```python
from build123d import *

# Parameters (mm, degrees)
F0_R         = 25
F1_DEPTH     = 60
F2_W         = 33.9622593881
F2_H         = 36.695571085
F3_DEPTH     = 25
F4_R         = 18.3477855425
F5_DEPTH     = 25.0000003725
F6_R         = 5
F8_T1_DEPTH  = 37.8584149398
F8_T6_ANGLE  = 94.4306250519
F8_T11_ANGLE = 94.4306250519
F8_T16_ANGLE = 94.4306250519
F8_T21_ANGLE = 47.2153125259
F8_T26_ANGLE = 47.2153125259
F8_T31_ANGLE = 47.2153125259
F8_T36_ANGLE = 47.2153125259
F8_T41_ANGLE = 85.5693749481
F8_T46_ANGLE = 85.5693749481
F8_T51_ANGLE = 85.5693749481
F8_T56_ANGLE = 85.5693749481
F8_T61_ANGLE = 85.5693749481
F8_T66_ANGLE = 85.5693749481
F9_R         = 14.0953649679
F10_DEPTH    = 200


# Not quite as in the source:
# - a fillet or chamfer that OpenCascade refuses, or shapes differently, is made with other operations: its cross-section is extruded or revolved along the edge and cut away or added
# - a feature of the source that left no trace in its solid (it failed there, or was rolled back) is left out


with BuildPart() as f1:
    # F0 (on Front) → F1 (new body)
    with BuildSketch(Plane.XZ):
        Circle(F0_R)
    extrude(amount=F1_DEPTH)

    # F2 (on face) → F3 (join)
    with BuildSketch(Plane.XZ.offset(60)):
        Rectangle(F2_W, F2_H)
    extrude(amount=F3_DEPTH)

    # F4 (on face) → F5 (join)
    with BuildSketch(Plane.XZ.offset(85)):
        Circle(F4_R)
    extrude(amount=F5_DEPTH)

    # F6
    f6_edges = [f1.edges().sort_by_distance(p)[0] for p in [
        (-18.347786, -110, 0),
    ]]
    fillet(f6_edges, radius=F6_R)

    # F8: chamfer of 5 on 9 edges, made by hand

    # F8_s2 → F8_t1 (cut)
    with BuildSketch(Plane.XZ.offset(60)):
        Polygon((16.9811296941, -13.3477855425), (11.9811296941, -18.3477855425), (16.9811296941, -18.3477855425), align=None)
        Polygon((16.9811296941, 13.3477855425), (11.9811296941, 18.3477855425), (16.9811296941, 18.3477855425), align=None)
        Polygon((-11.9811296941, -18.3477855425), (-16.9811296941, -13.3477855425), (-16.9811296941, -18.3477855425), align=None)
        Polygon((-16.9811296941, 13.3477855425), (-11.9811296941, 18.3477855425), (-16.9811296941, 18.3477855425), align=None)
    extrude(amount=F8_T1_DEPTH, mode=Mode.SUBTRACT)


with BuildPart() as f8_tool4:
    # F8_s5 → F8_t6 (revolve)
    with BuildSketch(Plane(origin=(0, 0, 0), x_dir=(0, 1, 0), z_dir=(0.7339114217, 0, 0.6792451878))):
        Polygon((-60, 20), (-55, 25), (-60, 25), align=None)
    revolve(axis=Axis((0, -60, 0), (0, -1, 0)), revolution_arc=F8_T6_ANGLE)

    split(bisect_by=Plane(origin=(-15.1644576183, 0, 15.1644576183), x_dir=(0, 1, 0), z_dir=(-0.7071067812, 0, 0.7071067812)), keep=Keep.TOP)


with BuildPart() as f1_1:
    add(f1.part)

    # F8_t3: cut F8_tool4
    add(f8_tool4.part, mode=Mode.SUBTRACT)


with BuildPart() as f8_tool9:
    # F8_s10 → F8_t11 (revolve)
    with BuildSketch(Plane(origin=(0, 0, 0), x_dir=(0, 1, 0), z_dir=(0.7339114217, 0, 0.6792451878))):
        Polygon((-60, 20), (-55, 25), (-60, 25), align=None)
    revolve(axis=Axis((0, -60, 0), (0, -1, 0)), revolution_arc=F8_T11_ANGLE)

    split(bisect_by=Plane.YZ.offset(-16.9811296941), keep=Keep.BOTTOM)


with BuildPart() as f1_2:
    add(f1_1.part)

    # F8_t8: cut F8_tool9
    add(f8_tool9.part, mode=Mode.SUBTRACT)


with BuildPart() as f8_tool14:
    # F8_s15 → F8_t16 (revolve)
    with BuildSketch(Plane(origin=(0, 0, 0), x_dir=(0, 1, 0), z_dir=(0.7339114217, 0, 0.6792451878))):
        Polygon((-60, 20), (-55, 25), (-60, 25), align=None)
    revolve(axis=Axis((0, -60, 0), (0, -1, 0)), revolution_arc=F8_T16_ANGLE)

    split(bisect_by=Plane(origin=(-15.1644576183, 0, -15.1644576183), x_dir=(0, 1, 0), z_dir=(-0.7071067812, 0, -0.7071067812)), keep=Keep.TOP)


with BuildPart() as f1_3:
    add(f1_2.part)

    # F8_t13: cut F8_tool14
    add(f8_tool14.part, mode=Mode.SUBTRACT)


with BuildPart() as f8_tool19:
    # F8_s20 → F8_t21 (revolve)
    with BuildSketch(Plane(origin=(0, 0, 0), x_dir=(0, 1, 0), z_dir=(-0.7339114217, 0, -0.6792451878))):
        Polygon((-60, 20), (-55, 25), (-60, 25), align=None)
    revolve(axis=Axis((0, -60, 0), (0, -1, 0)), revolution_arc=F8_T21_ANGLE)

    split(bisect_by=Plane(origin=(15.1644576183, 0, -15.1644576183), x_dir=(0, 1, 0), z_dir=(0.7071067812, 0, -0.7071067812)), keep=Keep.TOP)


with BuildPart() as f1_4:
    add(f1_3.part)

    # F8_t18: cut F8_tool19
    add(f8_tool19.part, mode=Mode.SUBTRACT)


with BuildPart() as f8_tool24:
    # F8_s25 → F8_t26 (revolve)
    with BuildSketch(Plane(origin=(0, 0, 0), x_dir=(0, 1, 0), z_dir=(-0.7339114217, 0, -0.6792451878))):
        Polygon((-60, 20), (-55, 25), (-60, 25), align=None)
    revolve(axis=Axis((0, -60, 0), (0, -1, 0)), revolution_arc=F8_T26_ANGLE)

    split(bisect_by=Plane.YZ.offset(16.9811296941), keep=Keep.TOP)


with BuildPart() as f1_5:
    add(f1_4.part)

    # F8_t23: cut F8_tool24
    add(f8_tool24.part, mode=Mode.SUBTRACT)


with BuildPart() as f8_tool29:
    # F8_s30 → F8_t31 (revolve)
    with BuildSketch(Plane.XY):
        Polygon((20, -60), (25, -55), (25, -60), align=None)
    revolve(axis=Axis((0, -60, 0), (0, -1, 0)), revolution_arc=F8_T31_ANGLE)

    split(bisect_by=Plane.YZ.offset(16.9811296941), keep=Keep.TOP)


with BuildPart() as f1_6:
    add(f1_5.part)

    # F8_t28: cut F8_tool29
    add(f8_tool29.part, mode=Mode.SUBTRACT)


with BuildPart() as f8_tool34:
    # F8_s35 → F8_t36 (revolve)
    with BuildSketch(Plane.XY):
        Polygon((20, -60), (25, -55), (25, -60), align=None)
    revolve(axis=Axis((0, -60, 0), (0, -1, 0)), revolution_arc=F8_T36_ANGLE)

    split(bisect_by=Plane(origin=(15.1644576183, 0, 15.1644576183), x_dir=(0, 1, 0), z_dir=(0.7071067812, 0, 0.7071067812)), keep=Keep.TOP)


with BuildPart() as f1_7:
    add(f1_6.part)

    # F8_t33: cut F8_tool34
    add(f8_tool34.part, mode=Mode.SUBTRACT)


with BuildPart() as f8_tool39:
    # F8_s40 → F8_t41 (revolve)
    with BuildSketch(Plane(origin=(0, 0, 0), x_dir=(0, 1, 0), z_dir=(-0.7339114217, 0, 0.6792451878))):
        Polygon((-60, 20), (-55, 25), (-60, 25), align=None)
    revolve(axis=Axis((0, -60, 0), (0, -1, 0)), revolution_arc=F8_T41_ANGLE)

    split(bisect_by=Plane(origin=(-15.1644576183, 0, -15.1644576183), x_dir=(0, 1, 0), z_dir=(-0.7071067812, 0, -0.7071067812)), keep=Keep.TOP)


with BuildPart() as f1_8:
    add(f1_7.part)

    # F8_t38: cut F8_tool39
    add(f8_tool39.part, mode=Mode.SUBTRACT)


with BuildPart() as f8_tool44:
    # F8_s45 → F8_t46 (revolve)
    with BuildSketch(Plane(origin=(0, 0, 0), x_dir=(0, 1, 0), z_dir=(-0.7339114217, 0, 0.6792451878))):
        Polygon((-60, 20), (-55, 25), (-60, 25), align=None)
    revolve(axis=Axis((0, -60, 0), (0, -1, 0)), revolution_arc=F8_T46_ANGLE)

    split(bisect_by=Plane.XY.offset(-18.3477855425), keep=Keep.BOTTOM)


with BuildPart() as f1_9:
    add(f1_8.part)

    # F8_t43: cut F8_tool44
    add(f8_tool44.part, mode=Mode.SUBTRACT)


with BuildPart() as f8_tool49:
    # F8_s50 → F8_t51 (revolve)
    with BuildSketch(Plane(origin=(0, 0, 0), x_dir=(0, 1, 0), z_dir=(-0.7339114217, 0, 0.6792451878))):
        Polygon((-60, 20), (-55, 25), (-60, 25), align=None)
    revolve(axis=Axis((0, -60, 0), (0, -1, 0)), revolution_arc=F8_T51_ANGLE)

    split(bisect_by=Plane(origin=(15.1644576183, 0, -15.1644576183), x_dir=(0, 1, 0), z_dir=(0.7071067812, 0, -0.7071067812)), keep=Keep.TOP)


with BuildPart() as f1_10:
    add(f1_9.part)

    # F8_t48: cut F8_tool49
    add(f8_tool49.part, mode=Mode.SUBTRACT)


with BuildPart() as f8_tool54:
    # F8_s55 → F8_t56 (revolve)
    with BuildSketch(Plane(origin=(0, 0, 0), x_dir=(0, 1, 0), z_dir=(0.7339114217, 0, -0.6792451878))):
        Polygon((-60, 20), (-55, 25), (-60, 25), align=None)
    revolve(axis=Axis((0, -60, 0), (0, -1, 0)), revolution_arc=F8_T56_ANGLE)

    split(bisect_by=Plane(origin=(15.1644576183, 0, 15.1644576183), x_dir=(0, 1, 0), z_dir=(0.7071067812, 0, 0.7071067812)), keep=Keep.TOP)


with BuildPart() as f1_11:
    add(f1_10.part)

    # F8_t53: cut F8_tool54
    add(f8_tool54.part, mode=Mode.SUBTRACT)


with BuildPart() as f8_tool59:
    # F8_s60 → F8_t61 (revolve)
    with BuildSketch(Plane(origin=(0, 0, 0), x_dir=(0, 1, 0), z_dir=(0.7339114217, 0, -0.6792451878))):
        Polygon((-60, 20), (-55, 25), (-60, 25), align=None)
    revolve(axis=Axis((0, -60, 0), (0, -1, 0)), revolution_arc=F8_T61_ANGLE)

    split(bisect_by=Plane.XY.offset(18.3477855425), keep=Keep.TOP)


with BuildPart() as f1_12:
    add(f1_11.part)

    # F8_t58: cut F8_tool59
    add(f8_tool59.part, mode=Mode.SUBTRACT)


with BuildPart() as f8_tool64:
    # F8_s65 → F8_t66 (revolve)
    with BuildSketch(Plane(origin=(0, 0, 0), x_dir=(0, 1, 0), z_dir=(0.7339114217, 0, -0.6792451878))):
        Polygon((-60, 20), (-55, 25), (-60, 25), align=None)
    revolve(axis=Axis((0, -60, 0), (0, -1, 0)), revolution_arc=F8_T66_ANGLE)

    split(bisect_by=Plane(origin=(-15.1644576183, 0, 15.1644576183), x_dir=(0, 1, 0), z_dir=(-0.7071067812, 0, 0.7071067812)), keep=Keep.TOP)


with BuildPart() as f1_13:
    add(f1_12.part)

    # F8_t63: cut F8_tool64
    add(f8_tool64.part, mode=Mode.SUBTRACT)

    # F9 (on face) → F10 (cut)
    with BuildSketch(Plane(origin=(0, 0, 0), x_dir=(-1, 0, 0), z_dir=(0, 1, 0))):
        with Locations((-0.2972558141, 0.1472756267)):
            Circle(F9_R)
    extrude(amount=-F10_DEPTH, mode=Mode.SUBTRACT)


solid = f1_13.part
```
Check sheet for the modelled part. Datum: model origin and axes. Units: mm. A direction names the side the tool comes from. Coordinates: 2 decimals unless noted, no trailing zeros. Order: outer loops, then holes, each group sorted by start corner. A loop starts at its lowest first (then second) coordinate and runs counter-clockwise, first axis right, second up. Notation, with made-up numbers: M 30.5,37.5 L 88.5,37.5 A7 ccw 88.5,43.5 Z; hole C -4,83 d8. An arc over 180 degrees is marked long. Write each question's results on one line, items separated by ' | '. Start each with the question number.
1. Mould release check, pull along Y, two halves, no side actions. Record for faces 6 (the face through (23.846, -27.115, 7.509)), 7 (the face through (11, 0, -11)), 8 (the face through (18, -60, 0)): +Y half, -Y half, draft (parallel to the pull), parting line (faces both ways), or undercut.
2. Access from +Z, -Z, +X, -X, +Y, -Y to the whole of each face (thin tool, end or side, straight path). Record for faces 1 (the face through (-14.45, -71.36, -15.88)), 2 (the face through (-14.52, -71.36, 15.81)), 3 (the face through (14.52, -71.36, 15.81)), 4 (the face through (-18, -60, 0)), 5 (the face through (14.52, -71.36, -15.81)).
3. Material ranges on probe 1 along Z at (x, y) = (6.5, -25.5); probe 2 along Y at (x, z) = (5, 21); probe 3 along Y at (x, z) = (-8, -17), recorded low to high.
4. Cross-section at B-B on y = -103. Record the cut outline in (x, z).
5. Cross-section at A-A on y = -62. Record the cut outline in (x, z).
6. Go/stop test with flat-tipped pins: P1, Ø5.5, axis at x = 11.5, z = -14.5, coming from the -Y side; P2, Ø1.8, axis at x = -2, z = 19.5, coming from the -Y side; P3, Ø1.5, axis at x = 18, z = -3, coming from the +Y side; P4, Ø3.5, axis at x = -10, z = -13, coming from the -Y side. Record where each tip stops, or that it passes through.
7. Cross-section at C-C on y = -7.5. Record the cut outline in (x, z), and give its area (3 significant figures).
Checks:
1) face 6: draft | face 7: +Y half | face 8: undercut
2) face 1: -Z, -X, -Y | face 2: +Z, -X, -Y | face 3: +Z, +X, -Y | face 4: +Z, -Z, -X | face 5: -Z, +X, -Y
3) probe 1: z = -24.14 to -12.51, 12.8 to 24.14 | probe 2: y = -58.41 to 0 | probe 3: y = -85 to 0
4) outline: C 0,0 d36.7; hole C 0.3,0.15 d28.19
5) outline: M -16.98,-13.35 L -11.98,-18.35 L 11.98,-18.35 L 16.98,-13.35 L 16.98,13.35 L 11.98,18.35 L -11.98,18.35 L -16.98,13.35 Z; hole C 0.3,0.15 d28.19
6) P1: stops at y = -109.38 | P2: stops at y = -60 | P3: stops at y = 0 | P4: stops at y = -109.83
7) outline: C 0,0 d50; hole C 0.3,0.15 d28.19 | area: 1,340 mm²
